Could you check a few things on this model? Use its own coordinates, in mm. A direction names the side the tool comes from. Coordinates: 2 decimals unless noted, no trailing zeros. Loops run counter-clockwise (first coordinate to the right, second up) from the corner with the lowest first, then second, coordinate; pieces in that order, holes last.
from build123d import *

# Parameters (mm, degrees)
SKETCH1_R             = 1.75
BOSS_EXTRUDE1_DEPTH   = 5
BOSS_EXTRUDE1_2_DEPTH = 5
SKETCH1_2_R           = 1.75
BOSS_EXTRUDE2_DEPTH   = 5
BOSS_EXTRUDE3_DEPTH   = 28
FILLET1_R             = 1.4


with BuildPart() as part:
    # Sketch1 → Boss-Extrude1 (new body)
    with BuildSketch(Plane.XY):
        Polygon((-3, 3), (5.1, 3), (5.1, -32), (-3, -32), (-3, -26), align=None)
        Circle(SKETCH1_R, mode=Mode.SUBTRACT)
        with Locations(Location((0, -29, 0), (0, 0, 180))):
            Circle(SKETCH1_R, mode=Mode.SUBTRACT)
    extrude(amount=BOSS_EXTRUDE1_DEPTH)



with BuildPart() as body_2:
    # Sketch1 → Boss-Extrude1 2 (new body)
    with BuildSketch(Plane.XY):
        Polygon((50.27, 3), (42.17, 3), (42.17, -32), (50.27, -32), (50.27, -26), align=None)
        with Locations((47.27, 0)):
            Circle(SKETCH1_R, mode=Mode.SUBTRACT)
        with Locations(Location((47.27, -29, 0), (0, 0, 180))):
            Circle(SKETCH1_R, mode=Mode.SUBTRACT)
    extrude(amount=BOSS_EXTRUDE1_2_DEPTH)


with BuildPart() as part_1:
    add(part.part)

    add(body_2.part)  # Boss-Extrude2 merges body 2
    # Sketch1_2 → Boss-Extrude2 (add)
    # profile 1 of 2: a face of its own
    with BuildSketch(Plane.XY):
        Polygon((-3, 3), (5.1, 3), (5.1, -32), (-3, -32), (-3, -26), align=None)
        Circle(SKETCH1_2_R, mode=Mode.SUBTRACT)
        with Locations(Location((0, -29, 0), (0, 0, 180))):
            Circle(SKETCH1_2_R, mode=Mode.SUBTRACT)
    # profile 2 of 2: a face of its own
    with BuildSketch(Plane.XY):
        Polygon((50.27, 3), (42.17, 3), (42.17, -32), (50.27, -32), (50.27, -26), align=None)
        with Locations((47.27, 0)):
            Circle(SKETCH1_2_R, mode=Mode.SUBTRACT)
        with Locations(Location((47.27, -29, 0), (0, 0, 180))):
            Circle(SKETCH1_2_R, mode=Mode.SUBTRACT)
    extrude(amount=BOSS_EXTRUDE2_DEPTH)

    # Sketch2 → Boss-Extrude3 (add)
    with BuildSketch(Plane(origin=(0, 3, 0), x_dir=(1, 0, 0), z_dir=(0, 1, 0))):
        with BuildLine():
            Line((42.17, 0), (44.305, 0))
            ThreePointArc((44.305, 0), (23.635, -20.235462541), (2.965, 0))
            Line((2.965, 0), (5.1, 0))
            ThreePointArc((5.1, 0), (23.635, -18.100999821), (42.17, 0))
        make_face()
    extrude(amount=-BOSS_EXTRUDE3_DEPTH)

    # Fillet1
    fillet1_edges = [part_1.edges().sort_by_distance(p)[0] for p in [
        (5.1, -28.5, 5),
        (42.17, -28.5, 5),
    ]]
    fillet(fillet1_edges, radius=FILLET1_R)


solid = part_1.part
(1) Imagine slicing it at A-A, the plane x = 0. Write out the boundary of the cut face in (y, z).
Answers:
outline: (-32, 0) - (-30.75, 0) - (-30.75, 5) - (-32, 5) - close; (-27.25, 0) - (-1.75, 0) - (-1.75, 5) - (-27.25, 5) - close; (1.75, 0) - (3, 0) - (3, 5) - (1.75, 5) - close
(2) For pin 1 (1 mm diameter, centred on y = -20.5, z = 7.5, fed in from +X); pin 2 (4 mm diameter, centred on x = 20, y = -3, fed in from +Z); pin 3 (3 mm diameter, centred on y = -23.5, z = 17.5, fed in from +X); pin 4 (2 mm diameter, centred on x = 47.27, y = -29, fed in from -Z), each with a flat end and sliding along its axis, tell me the tip position at first contact or that it passes through.
Answers:
pin 1: stops at x = 42.92
pin 2: stops at z = 20.17
pin 3: stops at x = 36.17
pin 4: passes through
(3) Imagine slicing it at C-C, the plane z = 3. Write out the boundary of the cut face in (x, y).
Answers:
outline: (-3, -32) - (5.1, -32) - (5.1, -25) - (5.42, -25) - (5.42, 3) - (-3, 3) - close; (41.85, -25) - (42.17, -25) - (42.17, -32) - (50.27, -32) - (50.27, 3) - (41.85, 3) - close; hole circle Ø3.5 at (0, -29); hole circle Ø3.5 at (0, 0); hole circle Ø3.5 at (47.27, -29); hole circle Ø3.5 at (47.27, 0)
(4) I need wall thicknesses on probe 1 along Y at (x, z) = (47.27, 4); probe 2 along X at (y, z) = (-29, 1.1); probe 3 along Z at (x, y) = (47, -25.5). Which ranges of each line are inside material? Lowest first, please.
Answers:
probe 1: y = -32 to -30.75, -27.25 to -1.75, 1.75 to 3
probe 2: x = -3 to -1.75, 1.75 to 5.1, 42.17 to 45.52, 49.02 to 50.27
probe 3: z = 0 to 5
(5) Which directions (+Z, -Z, +X, -X, +Y, -Y) give clear straight access to the entire face, cutting with the end or side of a thin tool? Please do faces 4 (the face through (0, -14, 5)), 5 (the face through (4.7, -28.55, 4.58)), 6 (the face through (47, -14, 5)), 7 (the face through (5.1, -28, 2)).
Answers:
face 4: +Z, -X, +Y, -Y
face 5: +Z, -Y
face 6: +Z, +X, +Y, -Y
face 7: +Z, -Z, -Y
(6) Imagine slicing it at B-B, the plane y = -29. Write out the boundary of the cut face in (x, z), and give its area (3 significant figures).
Answers:
outline: (-3, 0) - (-1.75, 0) - (-1.75, 5) - (-3, 5) - close; (1.75, 0) - (5.1, 0) - (5.1, 3.6) arc R1.4 ccw to (3.7, 5) - (1.75, 5) - close; (42.17, 0) - (45.52, 0) - (45.52, 5) - (43.57, 5) arc R1.4 ccw to (42.17, 3.6) - close; (49.02, 0) - (50.27, 0) - (50.27, 5) - (49.02, 5) - close
area: 45.2 mm2
(7) We'd pull the mould along Y, two halves only. Please class faces 1 (the face through (45.653, -28.33, 2.465)), 2 (the face through (23.7, -25, 18.3)), 3 (the face through (42.17, -28, 2)): +Y half, -Y half, draft (parallel to the pull), parting line (faces both ways), or undercut.
Answers:
face 1: undercut
face 2: -Y half
face 3: draft
(8) Imagine slicing it at D-D, the plane z = 17.25. Write out the boundary of the cut face in (x, y).
Answers:
outline: (12.93, -25) - (18.08, -25) - (18.08, 3) - (12.93, 3) - close; (29.19, -25) - (34.34, -25) - (34.34, 3) - (29.19, 3) - close
